from build123d import *

# Parameters (mm, degrees)
SZKIC1_W                    = 300
SZKIC1_H                    = 150
DODANIE_WYCI_GNI_CIE1_DEPTH = 10
SZKIC2_R                    = 5.25
WYTNIJ_WYCI_GNI_CIE1_DEPTH  = 2
ZAOKR_GLENIE1_R             = 15


with BuildPart() as part:
    # Szkic1 → Dodanie-wyciągnięcie1 (new body)
    with BuildSketch(Plane.XY):
        Rectangle(SZKIC1_W, SZKIC1_H)
    extrude(amount=DODANIE_WYCI_GNI_CIE1_DEPTH)

    # Szkic2 → Wytnij-wyciągnięcie1 (cut)
    with BuildSketch(Plane.XY.offset(10)):
        with Locations((-140, 0)):
            Circle(SZKIC2_R)
        with Locations((-42.5, 56.291651246)):
            Circle(SZKIC2_R)
        with Locations((-42.5, -56.291651246)):
            Circle(SZKIC2_R)
    extrude(amount=-WYTNIJ_WYCI_GNI_CIE1_DEPTH, mode=Mode.SUBTRACT)

    # Zaokrąglenie1
    zaokr_glenie1_edges = [part.edges().sort_by_distance(p)[0] for p in [
        (150, -75, 5),
        (-150, -75, 5),
        (-150, 75, 5),
        (150, 75, 5),
    ]]
    fillet(zaokr_glenie1_edges, radius=ZAOKR_GLENIE1_R)


solid = part.part
Geometry: final body of the model. Coordinates: model frame, mm. A direction names the side the tool comes from. Give positions to 0.01 mm unless a question says otherwise; leave off trailing zeros. Order: outer loops, then holes, each group sorted by start corner. A loop starts at its lowest first (then second) coordinate and runs counter-clockwise, first axis right, second up. Notation, with made-up numbers: (57.5, 10) -> (86.5, 10) arc R10 cw to (86.5, 21) -> close; hole circle Ø9 at (44.5, -12). An arc over 180 degrees is marked (long way). Write each question's results on one line, items separated by ' | '.
1) Draft query along Y for faces 1 (the face through (-43.183, 61.497, 9.014)), 2 (the face through (145.49, 70.72, 5.07)), 3 (the face through (-43, 56, 8)), 4 (the face through (-2, 1, 0)). Return one class per face: released by +Y, released by -Y, zero draft, split by the parting line, or undercut.
Geometry says:
face 1: undercut | face 2: released by +Y | face 3: undercut | face 4: zero draft
2) Line query: line 1 along Y through (x, z) = (-42.5, 8.45); line 2 along Y through (x, z) = (-140, 9.55). Output: solid intervals per line, ascending.
Geometry says:
line 1: y = -75 to -61.54, -51.04 to 51.04, 61.54 to 75 | line 2: y = -74.14 to -5.25, 5.25 to 74.14
3) Set-up query: faces 5 (the face through (145.49, -70.72, 5.07)), 6 (the face through (-135, 1.6, 9)). Return all of +Z, -Z, +X, -X, +Y, -Y with unobstructed straight access to the full face (end or side cutting, diameter ignored); none if empty.
Geometry says:
face 5: +Z, -Z, +X, -Y | face 6: +Z
4) Cut plane B-B (x = -140). Output: boundary loops of the cut face in (y, z), and give its area (3 significant figures).
Geometry says:
outline: (-74.14, 0) -> (74.14, 0) -> (74.14, 10) -> (5.25, 10) -> (5.25, 8) -> (-5.25, 8) -> (-5.25, 10) -> (-74.14, 10) -> close | area: 1,460 mm²
5) First-contact query: pin 1 Ø3 at (x, y) = (-44.5, 54.5) entering from +Z; pin 2 Ø11.5 at (x, y) = (-45, -57) entering from +Z. Flat tips, straight axial feed; report the tip coordinate or a pass-through.
Geometry says:
pin 1: stops at z = 8 | pin 2: stops at z = 10
6) Cut plane A-A (x = -42.5). Output: boundary loops of the cut face in (y, z), and give its area (3 significant figures).
Geometry says:
outline: (-75, 0) -> (75, 0) -> (75, 10) -> (61.54, 10) -> (61.54, 8) -> (51.04, 8) -> (51.04, 10) -> (-51.04, 10) -> (-51.04, 8) -> (-61.54, 8) -> (-61.54, 10) -> (-75, 10) -> close | area: 1,460 mm²
